from build123d import *

# Parameters (mm, degrees)
BOSS_EXTRUDE1_DEPTH = 9
SKETCH3_R           = 2
SKETCH3_W           = 7
SKETCH3_H           = 1
CUT_EXTRUDE4_DEPTH  = 8
SKETCH4_W           = 1
SKETCH4_H           = 3
CUT_EXTRUDE5_DEPTH  = 1
SKETCH5_R           = 2
CUT_EXTRUDE6_DEPTH  = 11


with BuildPart() as part:
    # Sketch2 → Boss-Extrude1 (new body)
    with BuildSketch(Plane(origin=(0, 0, 0), x_dir=(1, 0, 0), z_dir=(0, 1, 0))):
        Polygon((0, 0), (0, 12), (9, 12), (9, 9), (2, 9), (2, 3), (7, 3), (7, 0), align=None)
    extrude(amount=BOSS_EXTRUDE1_DEPTH)

    # Sketch3 → Cut-Extrude4 (cut)
    with BuildSketch(Plane.XY):
        Polygon((8.855862573, 6), (7, 6), (7, 4), (7, 2), (8.855862573, 2), align=None)
        with Locations((5, 4)):
            Circle(SKETCH3_R)
        with BuildLine():
            Line((7, 4), (7, 6))
            Line((7, 6), (5, 6))
            ThreePointArc((5, 6), (6.414213562, 5.414213562), (7, 4))
        make_face()
        with BuildLine():
            Line((7, 2), (7, 4))
            ThreePointArc((7, 4), (6.414213562, 2.585786438), (5, 2))
            Line((5, 2), (7, 2))
        make_face()
        with Locations((5.5, 8.5)):
            Rectangle(SKETCH3_W, SKETCH3_H)
    extrude(amount=-CUT_EXTRUDE4_DEPTH, mode=Mode.SUBTRACT)

    # Sketch4 → Cut-Extrude5 (cut)
    with BuildSketch(Plane(origin=(0, 9, 0), x_dir=(1, 0, 0), z_dir=(0, 1, 0))):
        with Locations((1.5, 6)):
            Rectangle(SKETCH4_W, SKETCH4_H)
    extrude(amount=-CUT_EXTRUDE5_DEPTH, mode=Mode.SUBTRACT)

    # Sketch5 → Cut-Extrude6 (cut)
    with BuildSketch(Plane.XY.offset(-9)):
        Polygon((9, 9), (2, 9), (2, 8), (5, 8), (9, 8), align=None)
        with Locations((5, 4)):
            Circle(SKETCH5_R)
        with BuildLine():
            Line((9, 4.000000022), (9, 8))
            Line((9, 8), (5, 8))
            ThreePointArc((5, 8), (7.828427117, 6.828427133), (9, 4.000000022))
        make_face()
        with BuildLine():
            Line((9, 0), (9, 4.000000022))
            ThreePointArc((9, 4.000000022), (7.828427133, 1.171572883), (5, 0))
            Line((5, 0), (9, 0))
        make_face()
    extrude(amount=-CUT_EXTRUDE6_DEPTH, mode=Mode.SUBTRACT)


solid = part.part
Work out the finished part from the listing and answer in its coordinate system (mm). A direction names the side the tool comes from. Give positions to 0.01 mm unless a question says otherwise; leave off trailing zeros. Order: outer loops, then holes, each group sorted by start corner. A loop starts at its lowest first (then second) coordinate and runs counter-clockwise, first axis right, second up. Notation, with made-up numbers: M -10,66 L 6,66 A6 cw 6,72 Z; hole C 64.5,69 d3. An arc over 180 degrees is marked long. Return JSON: item names as keys, results as strings.
Q1. Find section B-B, the plane y = 3. Write down the section's boundary in (x, z).
Answer below:
{"outline": "M 0,-12 L 3.27,-12 L 3.27,-9 L 2,-9 L 2,-3 L 3.27,-3 L 3.27,0 L 0,0 Z; M 6.73,-12 L 8.87,-12 L 8.87,-9 L 6.73,-9 Z"}
Q2. Find section D-D, the plane z = -5.5. Write down the section's boundary in (x, y), and give its area (3 significant figures).
Answer below:
{"outline": "M 0,0 L 2,0 L 2,8 L 1,8 L 1,9 L 0,9 Z", "area": "17.0 mm^2"}
Q3. Find the intervals of material crossed by line 1 along Y through (x, z) = (5, -10.45); line 2 along Z through (x, y) = (6, 0.75); line 3 along X through (y, z) = (3, -3.5), in increasing order. Write a range as [from, to].
Answer below:
{"line 1": "y = [0, 2], [6, 8]", "line 2": "z = [-12, -9], [-3, 0]", "line 3": "x = [0, 2]"}
Q4. The mould has two halves that part along Y. Classify faces 5 (the face through (3, 4, -1)), 6 (the face through (2.8, 3.9, -3)), 7 (the face through (3, 8, -10)): pulls with the +Y half, pulls with the -Y half, needs draft (parallel to the pull), parting line crosses it, or undercut.
Answer below:
{"face 5": "undercut", "face 6": "needs draft", "face 7": "pulls with the +Y half"}
Q5. Find section A-A, the plane x = 2.25. Write down the section's boundary in (y, z).
Answer below:
{"outline": "M 0,-12 L 8,-12 L 8,-9 L 0,-9 Z; M 0,-3 L 8,-3 L 8,0 L 0,0 Z"}
Q6. Each of these flat-tipped pins is pushed along its axis until it touches: pin 1 (2 mm diameter, centred on y = 1, z = -1.5, fed in from +X); pin 2 (1.5 mm diameter, centred on x = 5.5, z = -3.5, fed in from +Y); pin 3 (2 mm diameter, centred on x = 6, y = 3.5, fed in from +Z). Where does it stop, or does it pass through?
Answer below:
{"pin 1": "stops at x = 7", "pin 2": "stops at y = 8", "pin 3": "stops at z = -9"}
Q7. Find section C-C, the plane z = -10. Write down the section's boundary in (x, y).
Answer below:
{"outline": "M 0,0 L 5,0 A4 ccw 5,8 L 2,8 L 2,9 L 0,9 Z; hole C 5,4 d4"}
Q8. Which of the six approach directions +Z, -Z, +X, -X, +Y, -Y give full straight-line access (tool end or side, diameter ignored) to faces 1 (the face through (4, 8, -1)), 2 (the face through (6, 2, -1)), 3 (the face through (7, 3, -9)), 4 (the face through (1.5, 8.5, -7.5))?
Answer below:
{"face 1": "+Z, -Z, +X, +Y", "face 2": "+Z, +X", "face 3": "+X, +Y, -Y", "face 4": "+X, +Y"}
